Geometry: final body of the model. Coordinates: model frame, mm. A direction names the side the tool comes from. Coordinates: 2 decimals unless noted, no trailing zeros. Loops run counter-clockwise (first coordinate to the right, second up) from the corner with the lowest first, then second, coordinate; pieces in that order, holes last. Notation, with made-up numbers: (-24, 25) - (30, 25) arc R17 ccw to (30, 34) - close; hole circle Ø6 at (5, -18.75). An arc over 180 degrees is marked (long way). Return JSON: item names as keys, results as strings.
from build123d import *

# Parameters (mm, degrees)
SKETCH1_R           = 2.5
BOSS_EXTRUDE1_DEPTH = 5
BOSS_EXTRUDE2_START = -5
SKETCH2_R           = 2.5
BOSS_EXTRUDE2_DEPTH = 5
SKETCH3_R           = 3.75
CUT_EXTRUDE1_DEPTH  = 2.5


with BuildPart() as part:
    # Sketch1 → Boss-Extrude1 (new body)
    with BuildSketch(Plane(origin=(0, 0, 0), x_dir=(1, 0, 0), z_dir=(0, 1, 0))):
        with BuildLine():
            Line((0, 5), (22.5, 5))
            ThreePointArc((22.5, 5), (27.5, 0), (22.5, -5))
            Line((22.5, -5), (0, -5))
            ThreePointArc((0, -5), (-5, 0), (0, 5))
        make_face()
        with Locations(Location((0, 0, 0), (0, 0, 270))):
            Circle(SKETCH1_R, mode=Mode.SUBTRACT)
        with Locations(Location((22.5, 0, 0), (0, 0, 270))):
            Circle(SKETCH1_R, mode=Mode.SUBTRACT)
    extrude(amount=BOSS_EXTRUDE1_DEPTH)

    # Sketch2 → Boss-Extrude2 (add)
    with BuildSketch(Plane(origin=(0, 5, 0), x_dir=(1, 0, 0), z_dir=(0, 1, 0)).offset(BOSS_EXTRUDE2_START)):
        with BuildLine():
            Line((2.5, -4.330127019), (-16.985571585, -15.580127019))
            ThreePointArc((-16.985571585, -15.580127019), (-23.815698604, -13.75), (-21.985571585, -6.919872981))
            Line((-21.985571585, -6.919872981), (-2.5, 4.330127019))
            ThreePointArc((-2.5, 4.330127019), (4.330127019, 2.5), (2.5, -4.330127019))
        make_face()
        with Locations(Location((-19.485571585, -11.25, 0), (0, 0, 270))):
            Circle(SKETCH2_R, mode=Mode.SUBTRACT)
        with Locations(Location((0, 0, 0), (0, 0, 270))):
            Circle(SKETCH2_R, mode=Mode.SUBTRACT)
    extrude(amount=BOSS_EXTRUDE2_DEPTH)

    # Sketch3 → Cut-Extrude1 (cut)
    with BuildSketch(Plane(origin=(0, 5, 0), x_dir=(1, 0, 0), z_dir=(0, 1, 0))):
        with Locations(Location((22.5, 0, 0), (0, 0, 270))):
            Circle(SKETCH3_R)
        with Locations(Location((-19.485571585, -11.25, 0), (0, 0, 270))):
            Circle(SKETCH3_R)
    extrude(amount=-CUT_EXTRUDE1_DEPTH, mode=Mode.SUBTRACT)


solid = part.part
Item 1: Reachability of faces 1 (the face through (12, 2, 5)), 2 (the face through (18.84, 3.77, -0.81)), 3 (the face through (25, 1, 0)) from +Z, -Z, +X, -X, +Y, -Y: full face, straight path, thin tool, end or side. Return the list, or none.
Worked out:
{"face 1": "+Z, +X, +Y, -Y", "face 2": "+Y", "face 3": "+Y, -Y"}
Item 2: Ray query, probe 1 along X at (y, z) = (3, 0); probe 2 along X at (y, z) = (1.1, 1); probe 3 along Z at (x, y) = (22.5, 1.15). Return the intervals inside material, ascending. Write a range as from..to.
Worked out:
{"probe 1": "-10..-2.5, 2.5..18.75, 26.25..27.5", "probe 2": "-11.73..-2.29, 2.29..20.21, 24.79..27.4", "probe 3": "-5..-2.5, 2.5..5"}
Item 3: Section query A-A, the plane z = 0. Return loops of the section in (x, y), and give its area (3 significant figures).
Worked out:
{"outline": "(-10, 0) - (-2.5, 0) - (-2.5, 5) - (-10, 5) - close; (2.5, 0) - (20, 0) - (20, 2.5) - (18.75, 2.5) - (18.75, 5) - (2.5, 5) - close; (25, 0) - (27.5, 0) - (27.5, 5) - (26.25, 5) - (26.25, 2.5) - (25, 2.5) - close", "area": "131 mm^2"}
Item 4: First-contact query: pin 1 Ø6 at (x, z) = (22, -0.5) entering from +Y; pin 2 Ø1.5 at (x, y) = (16.5, 1.5) entering from +Z; pin 3 Ø1.5 at (y, z) = (3, 14) entering from -X. Flat tips, straight axial feed; report the tip coordinate or a pass-through.
Worked out:
{"pin 1": "y = 2.5", "pin 2": "z = 5", "pin 3": "x = -24.07"}
Item 5: Section query D-D, the plane z = 11.75. Return loops of the section in (x, y).
Worked out:
{"outline": "(-24.46, 0) - (-21.94, 0) - (-21.94, 2.5) - (-23.2, 2.5) - (-23.2, 5) - (-24.46, 5) - close; (-17.04, 0) - (-10.35, 0) - (-10.35, 5) - (-15.77, 5) - (-15.77, 2.5) - (-17.04, 2.5) - close"}
Item 6: Section query B-B, the plane y = 0.55. Return loops of the section in (x, z), and give its area (3 significant figures).
Worked out:
{"outline": "(-21.99, 6.92) - (-2.5, -4.33) arc R5 ccw to (0, -5) - (22.5, -5) arc R5 ccw to (22.5, 5) - (1.34, 5) - (-16.99, 15.58) arc R5 ccw to start; hole circle Ø5 at (-19.49, 11.25); hole circle Ø5 at (0, 0); hole circle Ø5 at (22.5, 0)", "area": "469 mm^2"}
Item 7: Mould query, pull axis X, two halves, no side actions, for faces 4 (the face through (-12.379, 2.465, 1.374)), 5 (the face through (-20, 2.5, 14)), 6 (the face through (-19.321, 3.768, 7.504)), 7 (the face through (-23.76, 2.465, 13.845)). Classes: +X half, -X half, draft (parallel to the pull), parting line (faces both ways), or undercut.
Worked out:
{"face 4": "-X half", "face 5": "undercut", "face 6": "undercut", "face 7": "parting line"}
Item 8: Section query C-C, the plane x = 3.5. Return loops of the section in (y, z), and give its area (3 significant figures).
Worked out:
{"outline": "(0, -5) - (5, -5) - (5, 5) - (0, 5) - close", "area": "50.0 mm^2"}
